Design review of the part built by this model. Coordinates are the model's own, in mm. Face numbers are marked on the shaded views. A direction names the side the tool comes from. Give positions to 0.01 mm unless a question says otherwise; leave off trailing zeros. Loops run counter-clockwise (first coordinate to the right, second up) from the corner with the lowest first, then second, coordinate; pieces in that order, holes last. Notation, with made-up numbers: (-16.5, 86.25) -> (0.5, 86.25) arc R24 cw to (0.5, 105.25) -> close; hole circle Ø10 at (18, -18.75). An arc over 180 degrees is marked (long way). Answer in a Markdown table with one row per item. Add a question column.
(1) Consider section A-A on z = 3. Write out the cut boundary in (x, y).
(2) Consider section B-B on y = 28.27. Write out the cut boundary in (x, z), then the cut area to 3 significant figures.
(3) For the marked faces 1, 2 and 3, list the 3-axis set-ups (+Z, -Z, +X, -X, +Y, -Y) from which the entire face can be reached by the end or side of a thin tool; tool diameter is ignored.
(4) For line 1 (Z direction, x = 51.5, y = 4); line 2 (Y direction, x = 68, z = 7.25); line 3 (X direction, y = 27, z = 5.75), list the stretches that pass through material, from the lowest coordinate up.
(5) For pin 1 (1 mm diameter, centred on y = 17.5, z = 4.5, fed in from +X); pin 2 (10 mm diameter, centred on x = 11.5, y = 1, fed in from -Z); pin 3 (1 mm diameter, centred on y = 26, z = 1, fed in from +X), all flat-tipped, find the tip position at first contact; note any pin that passes through.
(6) Consider section C-C on x = 78.5. Write out the cut boundary in (y, z), then the cut area to 3 significant figures.
(7) Consider section D-D on y = 16.5. Write out the cut boundary in (x, z), then the cut area to 3 significant figures.
from build123d import *

# Parameters (mm, degrees)
SKETCH_1_R      = 1.5
EXTRUDE_1_DEPTH = 10
FILLET_1_R      = 3
EXTRUDE_START   = -11
SKETCH_2_R      = 2.5
SKETCH_2_R_2    = 1.5
EXTRUDE_2_DEPTH = 11


with BuildPart() as part:
    # 草图1 → 凸台-拉伸1 (new body)
    with BuildSketch(Plane.XY):
        Polygon((-7.5, 4), (-7.5, -4), (7.5, -4), (15, 0), (70, 0), (116.765371804, 27), (113.301270189, 33), (70, 8), (0, 8), align=None)
        with Locations((112.0368731, 28.27)):
            Circle(SKETCH_1_R, mode=Mode.SUBTRACT)
        with Locations((70.727461339, 4.42)):
            Circle(SKETCH_1_R, mode=Mode.SUBTRACT)
    extrude(amount=EXTRUDE_1_DEPTH)

    # 圆角1
    fillet_1_edges = [part.edges().sort_by_distance(p)[0] for p in [
        (-7.5, 4, 5),
        (0, 8, 5),
        (70, 8, 5),
        (113.301270189, 33, 5),
        (116.765371804, 27, 5),
        (70, 0, 5),
        (15, 0, 5),
    ]]
    fillet(fillet_1_edges, radius=FILLET_1_R)

    # 草图2 → 凸台-拉伸2 (add)
    with BuildSketch(Plane.XY.offset(10).offset(EXTRUDE_START)):
        with Locations((112.0368731, 28.27)):
            Circle(SKETCH_2_R)
        with Locations((112.0368731, 28.27)):
            Circle(SKETCH_2_R_2, mode=Mode.SUBTRACT)
    extrude(amount=EXTRUDE_2_DEPTH)


solid = part.part
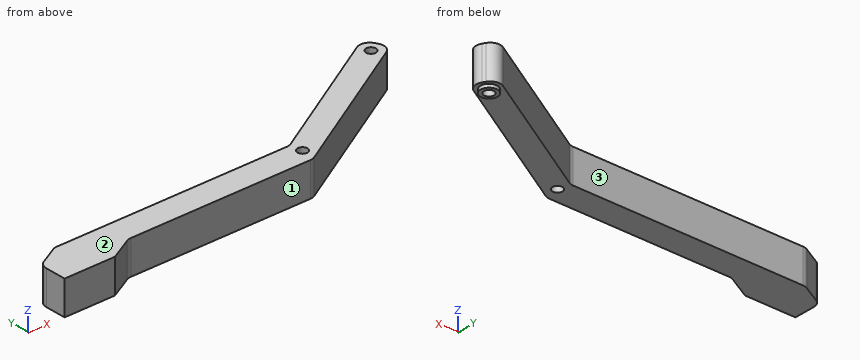
Values follow:
| question | item | result |
|---|---|---|
| 1 | outline | (-7.5, -4) -> (7.5, -4) -> (14.34, -0.35) arc R3 cw to (15.75, 0) -> (69.2, 0) arc R3 ccw to (70.7, 0.4) -> (114.17, 25.5) arc R3 ccw to (115.27, 29.6) -> (114.8, 30.4) arc R3 ccw to (110.7, 31.5) -> (70.7, 8.4) arc R3 cw to (69.2, 8) -> (0.75, 8) arc R3 ccw to (-0.66, 7.65) -> (-5.91, 4.85) arc R3 ccw to (-7.5, 2.2) -> close; hole circle Ø3 at (70.73, 4.42); hole circle Ø3 at (112.04, 28.27) |
| 2 | outline | (105.11, 0) -> (109.54, 0) -> (109.54, -1) -> (110.54, -1) -> (110.54, 10) -> (105.11, 10) -> close; (113.54, -1) -> (114.54, -1) -> (114.54, 0) -> (115.66, 0) -> (115.66, 10) -> (113.54, 10) -> close |
| 2 | area | 77.5 mm2 |
| 3 | face 1 | +Z, -Z, +X, -Y |
| 3 | face 2 | +Z, +X, -X, +Y, -Y |
| 3 | face 3 | +Z, -Z, -X, +Y |
| 4 | line 1 | 0 to 10 |
| 4 | line 2 | 0 to 8 |
| 4 | line 3 | 102.91 to 111.24, 112.84 to 115.46 |
| 5 | pin 1 | x = 101.18 |
| 5 | pin 2 | z = 0 |
| 5 | pin 3 | x = 115.21 |
| 6 | outline | (4.91, 0) -> (12.91, 0) -> (12.91, 10) -> (4.91, 10) -> close |
| 6 | area | 80.0 mm2 |
| 7 | outline | (84.72, 0) -> (98.58, 0) -> (98.58, 10) -> (84.72, 10) -> close |
| 7 | area | 139 mm2 |
